Answer from the drawing. Dimensions are ordinates in mm from the lowest x, y and z of the part. Coordinates: 2 decimals unless noted, no trailing zeros. Write each loop counter-clockwise with the first axis right and the second up, starting at its lowest first coordinate (ties: lowest second). Pieces come first, ordered by that corner, then holes. Notation, with made-up numbers: (83, 89.25) -> (88, 89.25) arc R16 cw to (88, 112.25) -> close; hole circle Ø6 at (-11, -11). An arc over 180 degrees is marked (long way). Return JSON: item names as keys, results as strings.
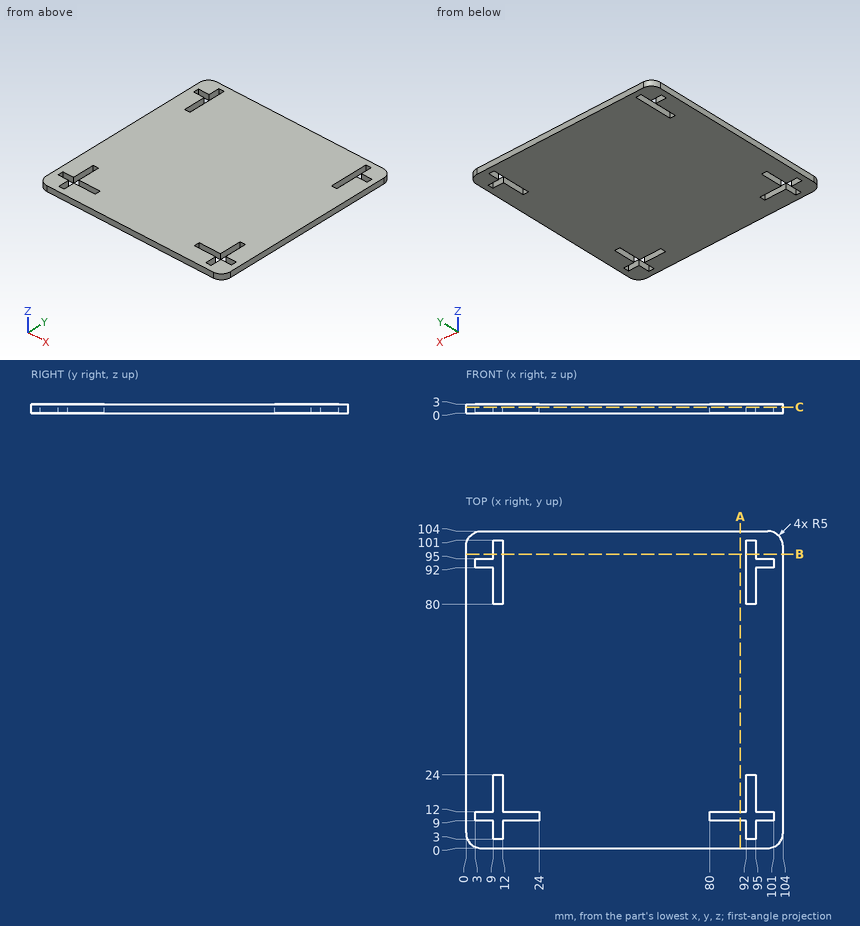
1. The part is cut by section C-C (z = 1.95). Count the separate pieces of the cut face and the enclosed holes in it, then the cut area to 3 significant figures.
Taken from the geometry:
{"separate pieces": "1", "enclosed holes": "4", "area": "10,400 mm2"}
2. The part is cut by section A-A (x = 90). Determine the outline of the cut face in (y, z).
Taken from the geometry:
{"outline": "(0, 0) -> (9, 0) -> (9, 3) -> (0, 3) -> close; (12, 0) -> (104, 0) -> (104, 3) -> (12, 3) -> close"}
3. The part is cut by section B-B (y = 96.5). Determine the outline of the cut face in (x, z), then the cut area to 3 significant figures.
Taken from the geometry:
{"outline": "(0, 0) -> (9, 0) -> (9, 3) -> (0, 3) -> close; (12, 0) -> (92, 0) -> (92, 3) -> (12, 3) -> close; (95, 0) -> (104, 0) -> (104, 3) -> (95, 3) -> close", "area": "294 mm2"}
4. A flat-ended cylindrical pin translates along its axis: pin 1 Ø1.5 at (x, z) = (59.5, 1) entering from -Y. Find the tip coordinate at first contact, or state that the pin passes through.
Taken from the geometry:
{"pin 1": "stops at y = 0"}
5. Consider L1, parallel to Y at x = 97.5, z = 2.4; L2, parallel to Y at x = 20, z = 0.6. Determine where each line is inside the solid, lowest interval first.
Taken from the geometry:
{"L1": "y = 0 to 9, 12 to 92, 95 to 104", "L2": "y = 0 to 9, 12 to 104"}
